Read the model definition and answer for the solid it produces. Units are mm, in the model's axes. A direction names the side the tool comes from. Give positions to 0.01 mm unless a question says otherwise; leave off trailing zeros. Loops run counter-clockwise (first coordinate to the right, second up) from the corner with the lowest first, then second, coordinate; pieces in that order, holes last. Notation, with made-up numbers: (17.25, 53) - (69.25, 53) arc R31 ccw to (69.25, 78) - close; hole circle Ø5 at (14, 41.5). An arc over 180 degrees is marked (long way). Use a Markdown table: item, result. Add a question column.
Item 1: Which of the six approach directions +Z, -Z, +X, -X, +Y, -Y give full straight-line access (tool end or side, diameter ignored) to faces 1 (the face through (6.46, 4, 11.62)), 2 (the face through (1.12, 4, 6.24)), 3 (the face through (0, 38, 12)), 4 (the face through (6, 1, 6)), 5 (the face through (44.451, -1, 6))?
Item 2: Consider probe 1 along Y at (x, z) = (3.5, 2.75); probe 2 along Y at (x, z) = (-23, 3.5); probe 3 along Z at (x, y) = (38, -1). Determine where each line is inside the solid, lowest interval first. Write a range as [from, to].
Item 3: A cutting plane is placed at C-C (z = 8). Determine the outline of the cut face in (x, y).
Item 4: A cutting plane is placed at B-B (x = 38.1). Determine the outline of the cut face in (y, z), plus the area to 4 significant figures.
Item 5: A cutting plane is placed at D-D (x = 23.5). Determine the outline of the cut face in (y, z).
Item 6: A cutting plane is placed at A-A (y = 53). Determine the outline of the cut face in (x, z).
Item 7: For a pull along Y with two mould halves and no side action, classify faces 6 (the face through (7, -3, 6)), 7 (the face through (6.46, 4, 1.12)), 8 (the face through (6.24, 66.1, 1.12)), 9 (the face through (12, 47, 0)) as +Y half, -Y half, draft (parallel to the pull), parting line (faces both ways), or undercut.
Item 8: Each of these flat-tipped pins is pushed along its axis until it touches: P1, Ø5, axis at x = 38.1, z = 6.35, coming from the -Y side (3 decimals); P2, Ø5, axis at y = 34.5, z = 3, coming from the -X side; P3, Ø0.7, axis at y = 24, z = 0.5, coming from the +X side; P4, Ø6, axis at x = 6.39, z = 6.35, coming from the +Y side. Where does it stop, or does it pass through?
from build123d import *

# Parameters (mm, degrees)
SKETCH1_W           = 12.7
SKETCH1_H           = 76.2
BOSS_EXTRUDE1_DEPTH = 12.7
SKETCH4_W           = 76.2
SKETCH4_H           = 12.7
BOSS_EXTRUDE3_DEPTH = 3
CUT_EXTRUDE5_DEPTH  = 12.7
CUT_EXTRUDE6_DEPTH  = 12.7
SKETCH16_R          = 5
CUT_EXTRUDE8_DEPTH  = 75.2
SKETCH17_R          = 3.175
CUT_EXTRUDE9_DEPTH  = 3
SKETCH18_R          = 3.175
CUT_EXTRUDE10_DEPTH = 3


with BuildPart() as part:
    # Sketch1 → Boss-Extrude1 (new body)
    with BuildSketch(Plane.XY):
        with Locations((6.35, 38.1)):
            Rectangle(SKETCH1_W, SKETCH1_H)
    extrude(amount=BOSS_EXTRUDE1_DEPTH)

    # Sketch4 → Boss-Extrude3 (add)
    with BuildSketch(Plane(origin=(0, 0, 0), x_dir=(-1, 0, 0), z_dir=(0, -1, 0))):
        with Locations((-6.351309366, -6.3465887)):
            Rectangle(SKETCH4_W, SKETCH4_H)
    extrude(amount=BOSS_EXTRUDE3_DEPTH)

    # Sketch12 → Cut-Extrude5 (cut)
    with BuildSketch(Plane.XY.offset(12.7)):
        with BuildLine():
            Line((1.35, 9), (1.35, 61.1))
            ThreePointArc((1.35, 61.1), (6.35, 66.1), (11.35, 61.1))
            Line((11.35, 61.1), (11.35, 9))
            ThreePointArc((11.35, 9), (6.35, 4), (1.35, 9))
        make_face()
    extrude(amount=-CUT_EXTRUDE5_DEPTH, mode=Mode.SUBTRACT)

    # Sketch13 → Cut-Extrude6 (cut)
    with BuildSketch(Plane(origin=(12.7, 0, 0), x_dir=(0, 0, -1), z_dir=(1, 0, 0))):
        with BuildLine():
            Line((-11.35, 9), (-11.35, 61.1))
            ThreePointArc((-11.35, 61.1), (-6.35, 66.1), (-1.35, 61.1))
            Line((-1.35, 61.1), (-1.35, 9))
            ThreePointArc((-1.35, 9), (-6.35, 4), (-11.35, 9))
        make_face()
    extrude(amount=-CUT_EXTRUDE6_DEPTH, mode=Mode.SUBTRACT)

    # Sketch16 → Cut-Extrude8 (cut)
    with BuildSketch(Plane(origin=(0, 76.2, 0), x_dir=(1, 0, 0), z_dir=(0, 1, 0))):
        with Locations(Location((6.394331047, -6.34829435, 0), (0, 0, 270))):
            Circle(SKETCH16_R)
    extrude(amount=-CUT_EXTRUDE8_DEPTH, mode=Mode.SUBTRACT)

    # Sketch17 → Cut-Extrude9 (cut)
    with BuildSketch(Plane(origin=(0, 0, 0), x_dir=(1, 0, 0), z_dir=(0, 1, 0))):
        with Locations(Location((-25.398690634, -6.3465887, 0), (0, 0, 270))):
            Circle(SKETCH17_R)
    extrude(amount=-CUT_EXTRUDE9_DEPTH, mode=Mode.SUBTRACT)

    # Sketch18 → Cut-Extrude10 (cut)
    with BuildSketch(Plane(origin=(0, 0, 0), x_dir=(1, 0, 0), z_dir=(0, 1, 0))):
        with Locations(Location((38.1, -6.3465887, 0), (0, 0, 270))):
            Circle(SKETCH18_R)
    extrude(amount=-CUT_EXTRUDE10_DEPTH, mode=Mode.SUBTRACT)


solid = part.part
Geometry says:
| question | item | result |
|---|---|---|
| 1 | face 1 | +Z, -Z |
| 1 | face 2 | +X, -X |
| 1 | face 3 | +Z, -Z, -X, +Y |
| 1 | face 4 | +Y |
| 1 | face 5 | +Z, -Z, +X, +Y, -Y |
| 2 | probe 1 | [-3, 1] |
| 2 | probe 2 | [-3, 0] |
| 2 | probe 3 | [0, 3.17], [9.52, 12.7] |
| 3 | outline | (-31.75, -3) - (-28.11, -3) - (-28.11, 0) - (-31.75, 0) - close; (-22.69, -3) - (35.39, -3) - (35.39, 0) - (12.7, 0) - (12.7, 4.28) - (11.11, 4.28) - (11.11, 1) - (1.68, 1) - (1.68, 4.28) - (0, 4.28) - (0, 0) - (-22.69, 0) - close; (0, 65.82) - (1.68, 65.82) - (1.68, 76.2) - (0, 76.2) - close; (11.11, 65.82) - (12.7, 65.82) - (12.7, 76.2) - (11.11, 76.2) - close; (40.81, -3) - (44.45, -3) - (44.45, 0) - (40.81, 0) - close |
| 4 | outline | (-3, 0) - (0, 0) - (0, 3.17) - (-3, 3.17) - close; (-3, 9.52) - (0, 9.52) - (0, 12.7) - (-3, 12.7) - close |
| 4 | area | 19.05 mm² |
| 5 | outline | (-3, 0) - (0, 0) - (0, 12.7) - (-3, 12.7) - close |
| 6 | outline | (0, 0) - (1.35, 0) - (1.35, 1.35) - (0, 1.35) - close; (0, 11.35) - (1.35, 11.35) - (1.35, 12.7) - (0, 12.7) - close; (11.35, 0) - (12.7, 0) - (12.7, 1.35) - (11.35, 1.35) - close; (11.35, 11.35) - (12.7, 11.35) - (12.7, 12.7) - (11.35, 12.7) - close |
| 7 | face 6 | -Y half |
| 7 | face 7 | undercut |
| 7 | face 8 | undercut |
| 7 | face 9 | draft |
| 8 | P1 | through |
| 8 | P2 | x = 0 |
| 8 | P3 | x = 12.7 |
| 8 | P4 | y = 1 |
